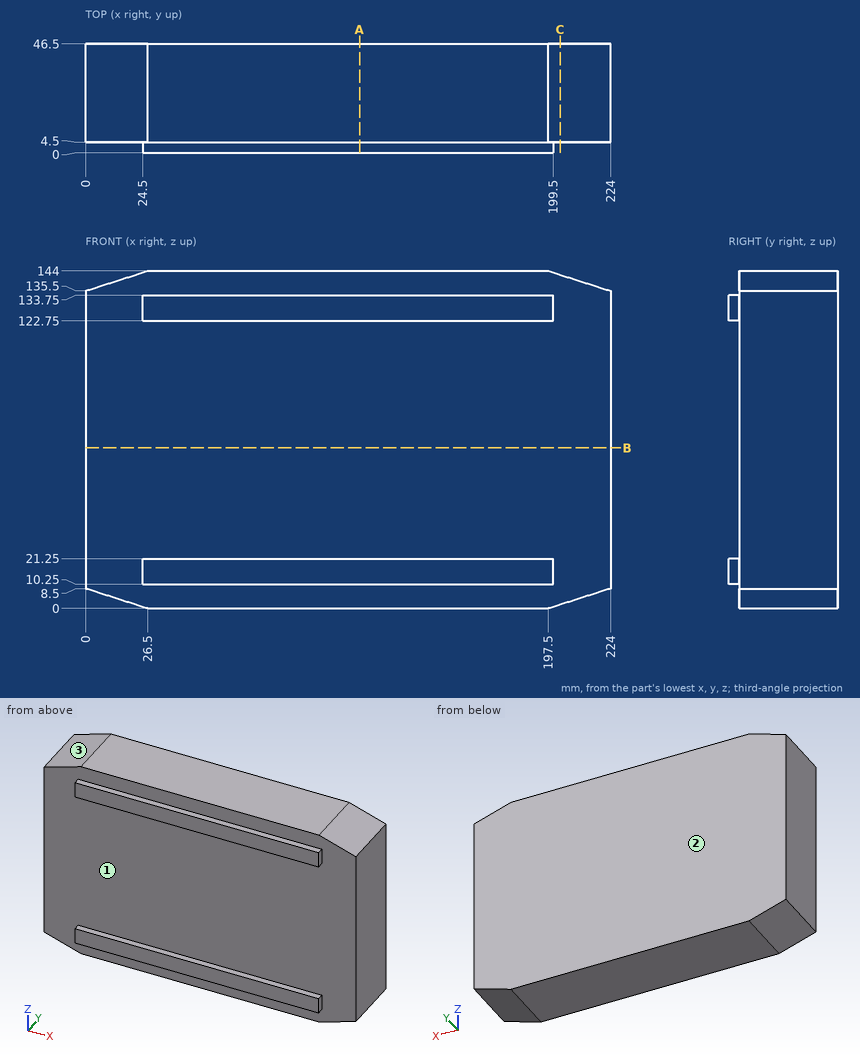
Can you work these out from the drawing? Everything is in mm from the part's minimum corner. Round coordinates to 2 decimals unless told otherwise and drop trailing zeros. Loops run counter-clockwise (first coordinate to the right, second up) from the corner with the lowest first, then second, coordinate; pieces in that order, holes last. Notation, with made-up numbers: (40, 34) -> (88, 34) arc R30 cw to (88, 56) -> close; hole circle Ø11 at (-12.5, 66). An arc over 180 degrees is marked (long way). Use CSV: the item, a comma, the result in double quotes.
(1) Suppose I cut it at A-A on x = 117. Write out the boundary of the cut face in (y, z), plus the area to 3 significant figures.
Return value:
outline,"(0, 10.25) -> (4.5, 10.25) -> (4.5, 0) -> (46.5, 0) -> (46.5, 144) -> (4.5, 144) -> (4.5, 133.75) -> (0, 133.75) -> (0, 122.75) -> (4.5, 122.75) -> (4.5, 21.25) -> (0, 21.25) -> close"
area,"6,150 mm²"
(2) If I drill on probe 1 along Z at (x, y) = (131, 4); probe 2 along Y at (x, z) = (38, 84.5); probe 3 along Z at (x, y) = (205, 14), over which ranges is the centre line in solid material (lowest first)? Write a range as [from, to].
Return value:
probe 1,"z = [10.25, 21.25], [122.75, 133.75]"
probe 2,"y = [4.5, 46.5]"
probe 3,"z = [2.41, 141.59]"
(3) If we mould it in two halves opening along Z, with no side actions, what happens to the marked faces 1, 2 and 3? For each: +Z half, -Z half, draft (parallel to the pull), parting line (faces both ways), or undercut.
Return value:
face 1,"undercut"
face 2,"draft"
face 3,"+Z half"
(4) Will these pins go through, and if not, where does the flat tip stop? pin 1 Ø1.3 at (x, y) = (155.5, 3) entering from +Z; pin 2 Ø4 at (x, z) = (180, 118) entering from -Y; pin 3 Ø3.5 at (x, y) = (110, 3) entering from -Z; pin 4 Ø2 at (x, y) = (103, 2) entering from -Z.
Return value:
pin 1,"stops at z = 133.75"
pin 2,"stops at y = 4.5"
pin 3,"stops at z = 0"
pin 4,"stops at z = 10.25"
(5) Suppose I cut it at C-C on x = 202.5. Write out the boundary of the cut face in (y, z).
Return value:
outline,"(4.5, 1.6) -> (46.5, 1.6) -> (46.5, 142.4) -> (4.5, 142.4) -> close"
(6) Suppose I cut it at B-B on z = 68.5. Write out the boundary of the cut face in (x, y).
Return value:
outline,"(0, 4.5) -> (224, 4.5) -> (224, 46.5) -> (0, 46.5) -> close"
